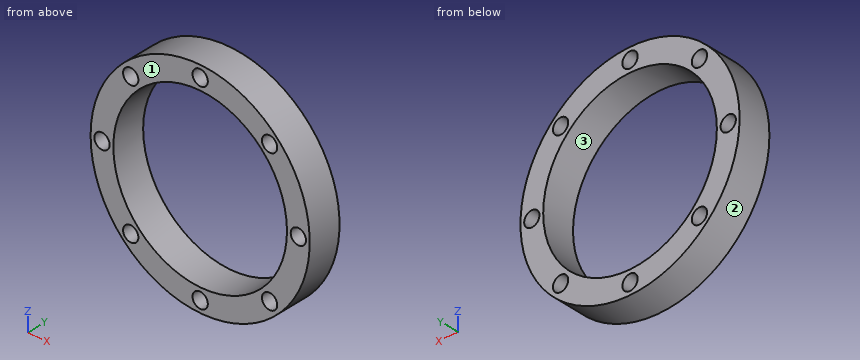
Autodesk Inventor part; units mm, degrees
ref_plane "YZ Plane" through (0, 0, 0) normal (1, 0, 0) x (0, 1, 0)
ref_plane "XZ Plane" through (0, 0, 0) normal (0, 1, 0) x (-1, 0, 0)
ref_plane "XY Plane" through (0, 0, 0) normal (0, 0, 1) x (1, 0, 0)
sketch "Szkic1" plane through (0, 0, 0) normal (0, 1, 0) x (-1, 0, 0)
  circle A0 centre (0, 0) radius 21
  circle A1 centre (0, 0) radius 26.5
  circle A2 centre (16.7938, 16.7938) radius 1.85
  circle A3 centre (0, 23.75) radius 1.85
  circle A4 centre (-16.7938, 16.7938) radius 1.85
  circle A5 centre (-23.75, 0) radius 1.85
  circle A6 centre (-16.7938, -16.7938) radius 1.85
  circle A7 centre (0, -23.75) radius 1.85
  circle A8 centre (16.7938, -16.7938) radius 1.85
  circle A9 centre (23.75, 0) radius 1.85
  line L0 (0, 21) -> (0, 26.5)
  dimension "d0" = 42
  dimension "d8" = 53
  dimension "d1" = 3.7
  dimension "d4" = 360
extrude "Wyciągnięcie proste1" add sketch "Szkic1" along normal blind 8
properties part number "Bell_KoloFormaGora"
The listing builds one solid part. Answer for the finished solid, in the listing's coordinates (mm). Face numbers are marked on the shaded views. Give positions to 0.01 mm unless a question says otherwise; leave off trailing zeros. Order: outer loops, then holes, each group sorted by start corner. A loop starts at its lowest first (then second) coordinate and runs counter-clockwise, first axis right, second up. Notation, with made-up numbers: (-31.75, 81) - (17.25, 81) arc R14 ccw to (17.25, 96) - close; hole circle Ø4 at (-28, 29). An arc over 180 degrees is marked (long way). Answer in a Markdown table with one row per item. Add a question column.
Q1. The part is cut by section A-A (x = 0). Determine the outline of the cut face in (y, z), then the cut area to 3 significant figures.
Q2. For a pull along Z with two mould halves and no side action, classify the marked faces 1, 2 and 3 as released by +Z, released by -Z, zero draft, split by the parting line, or undercut.
Q3. Find the intervals of material crossed by line 1 along Z through (x, y) = (0, 3.75); line 2 along X through (y, z) = (1.25, -1.5); line 3 along Z through (x, y) = (0.5, 7.5), in increasing order. Write a range as [from, to].
Q4. The part is cut by section D-D (x = -23.75). Determine the outline of the cut face in (y, z), then the cut area to 3 significant figures.
Q5. Given P1, Ø4, axis at y = 1.5, z = -15, coming from the -X side; P2, Ø1.5, axis at y = 3, z = -20, coming from the -X side, each flat-ended and moving along its own axis, determine where each tip first touches the part or whether it passes through.
Q6. The part is cut by section B-B (z = -23.75). Determine the outline of the cut face in (x, y).
Q7. The part is cut by section C-C (y = 5.5). Give the number of separate pieces and of enclosed holes in the cut face, then the cut area to 3 significant figures.
Determined:
| question | item | result |
|---|---|---|
| 1 | outline | (0, -26.5) - (8, -26.5) - (8, -25.6) - (0, -25.6) - close; (0, -21.9) - (8, -21.9) - (8, -21) - (0, -21) - close; (0, 21) - (8, 21) - (8, 21.9) - (0, 21.9) - close; (0, 25.6) - (8, 25.6) - (8, 26.5) - (0, 26.5) - close |
| 1 | area | 28.8 mm² |
| 2 | face 1 | zero draft |
| 2 | face 2 | split by the parting line |
| 2 | face 3 | undercut |
| 3 | line 1 | z = [-26.5, -25.6], [-21.9, -21], [21, 21.9], [25.6, 26.5] |
| 3 | line 2 | x = [-26.46, -24.83], [-22.67, -20.95], [20.95, 22.67], [24.83, 26.46] |
| 3 | line 3 | z = [-26.5, -25.53], [-21.97, -20.99], [20.99, 21.97], [25.53, 26.5] |
| 4 | outline | (0, -11.76) - (8, -11.76) - (8, -1.85) - (0, -1.85) - close; (0, 1.85) - (8, 1.85) - (8, 11.76) - (0, 11.76) - close |
| 4 | area | 158 mm² |
| 5 | P1 | stops at x = -23.09 |
| 5 | P2 | stops at x = -18.21 |
| 6 | outline | (-11.76, 0) - (-1.85, 0) - (-1.85, 8) - (-11.76, 8) - close; (1.85, 0) - (11.76, 0) - (11.76, 8) - (1.85, 8) - close |
| 7 | separate pieces | 1 |
| 7 | enclosed holes | 9 |
| 7 | area | 735 mm² |
